The listing builds one solid part. Answer for the finished solid, in the listing's coordinates (mm). Give positions to 0.01 mm unless a question says otherwise; leave off trailing zeros. Order: outer loops, then holes, each group sorted by start corner. A loop starts at its lowest first (then second) coordinate and runs counter-clockwise, first axis right, second up. Notation, with made-up numbers: (-5.75, 81.25) - (4.25, 81.25) arc R13 ccw to (4.25, 94.25) - close; hole circle Ø3 at (-26, 62.5). An arc over 180 degrees is marked (long way). Answer in a Markdown table with one row per item.
from build123d import *

# Parameters (mm, degrees)
SKETCH_1_W      = 260
SKETCH_1_H      = 120
SKETCH_1_R      = 1.8
SKETCH_1_R_2    = 11.5
SKETCH_1_R_3    = 1.75
SKETCH_1_W_2    = 10
SKETCH_1_H_2    = 30.9
SKETCH_1_W_3    = 6
SKETCH_1_H_3    = 6
EXTRUDE_1_DEPTH = 2


with BuildPart() as part:
    # 草圖1 → 填料-伸長1 (new body)
    with BuildSketch(Plane(origin=(0, 0, 0), x_dir=(1, 0, 0), z_dir=(0, 1, 0))):
        Rectangle(SKETCH_1_W, SKETCH_1_H)
        with Locations((-45, -9.55)):
            Circle(SKETCH_1_R, mode=Mode.SUBTRACT)
        with Locations((-45, -40.45)):
            Circle(SKETCH_1_R, mode=Mode.SUBTRACT)
        with Locations((30, -9.55)):
            Circle(SKETCH_1_R, mode=Mode.SUBTRACT)
        with Locations((30, -40.45)):
            Circle(SKETCH_1_R, mode=Mode.SUBTRACT)
        with Locations((95, -25)):
            Circle(SKETCH_1_R_2, mode=Mode.SUBTRACT)
        with Locations((-122, 52)):
            Circle(SKETCH_1_R_3, mode=Mode.SUBTRACT)
        with Locations((-122, -52)):
            Circle(SKETCH_1_R_3, mode=Mode.SUBTRACT)
        with Locations((122, 52)):
            Circle(SKETCH_1_R_3, mode=Mode.SUBTRACT)
        with Locations((122, -52)):
            Circle(SKETCH_1_R_3, mode=Mode.SUBTRACT)
        with Locations((-115, -17.5)):
            Circle(SKETCH_1_R, mode=Mode.SUBTRACT)
        with Locations((-115, -32.5)):
            Circle(SKETCH_1_R, mode=Mode.SUBTRACT)
        with Locations((-70, -25)):
            Rectangle(SKETCH_1_W_2, SKETCH_1_H_2, mode=Mode.SUBTRACT)
        with Locations((55, -50)):
            Rectangle(SKETCH_1_W_3, SKETCH_1_H_3, mode=Mode.SUBTRACT)
        with Locations((55, 0)):
            Rectangle(SKETCH_1_W_3, SKETCH_1_H_3, mode=Mode.SUBTRACT)
        with BuildLine():
            Line((-71.710967932, 42.596685205), (-69.210967932, 42.596685205))
            Line((-69.210967932, 42.596685205), (-69.210967932, 37.901740315))
            ThreePointArc((-69.210967932, 37.901740315), (-70.460967932, 22), (-71.710967932, 37.901740315))
            Line((-71.710967932, 37.901740315), (-71.710967932, 42.596685205))
        make_face(mode=Mode.SUBTRACT)
        with BuildLine():
            Line((-99.710967932, 42.596685205), (-97.210967932, 42.596685205))
            Line((-97.210967932, 42.596685205), (-97.210967932, 37.901740315))
            ThreePointArc((-97.210967932, 37.901740315), (-98.460967932, 22), (-99.710967932, 37.901740315))
            Line((-99.710967932, 37.901740315), (-99.710967932, 42.596685205))
        make_face(mode=Mode.SUBTRACT)
        with BuildLine():
            Line((-43.710967932, 42.596685205), (-41.210967932, 42.596685205))
            Line((-41.210967932, 42.596685205), (-41.210967932, 37.901740315))
            ThreePointArc((-41.210967932, 37.901740315), (-42.460967932, 22), (-43.710967932, 37.901740315))
            Line((-43.710967932, 37.901740315), (-43.710967932, 42.596685205))
        make_face(mode=Mode.SUBTRACT)
        with BuildLine():
            Line((-15.710967932, 42.596685205), (-13.210967932, 42.596685205))
            Line((-13.210967932, 42.596685205), (-13.210967932, 37.901740315))
            ThreePointArc((-13.210967932, 37.901740315), (-14.460967932, 22), (-15.710967932, 37.901740315))
            Line((-15.710967932, 37.901740315), (-15.710967932, 42.596685205))
        make_face(mode=Mode.SUBTRACT)
        with BuildLine():
            Line((12.289032068, 42.596685205), (14.789032068, 42.596685205))
            Line((14.789032068, 42.596685205), (14.789032068, 37.901740315))
            ThreePointArc((14.789032068, 37.901740315), (13.539032068, 22), (12.289032068, 37.901740315))
            Line((12.289032068, 37.901740315), (12.289032068, 42.596685205))
        make_face(mode=Mode.SUBTRACT)
        with BuildLine():
            Line((40.289032068, 42.596685205), (42.789032068, 42.596685205))
            Line((42.789032068, 42.596685205), (42.789032068, 37.901740315))
            ThreePointArc((42.789032068, 37.901740315), (41.539032068, 22), (40.289032068, 37.901740315))
            Line((40.289032068, 37.901740315), (40.289032068, 42.596685205))
        make_face(mode=Mode.SUBTRACT)
        with BuildLine():
            Line((68.289032068, 42.596685205), (70.789032068, 42.596685205))
            Line((70.789032068, 42.596685205), (70.789032068, 37.901740315))
            ThreePointArc((70.789032068, 37.901740315), (69.539032068, 22), (68.289032068, 37.901740315))
            Line((68.289032068, 37.901740315), (68.289032068, 42.596685205))
        make_face(mode=Mode.SUBTRACT)
        with BuildLine():
            Line((96.289032068, 42.596685205), (98.789032068, 42.596685205))
            Line((98.789032068, 42.596685205), (98.789032068, 37.901740315))
            ThreePointArc((98.789032068, 37.901740315), (97.539032068, 22), (96.289032068, 37.901740315))
            Line((96.289032068, 37.901740315), (96.289032068, 42.596685205))
        make_face(mode=Mode.SUBTRACT)
    extrude(amount=EXTRUDE_1_DEPTH)


solid = part.part
Item 1: Consider line 1 (X direction, y = 0.85, z = 52); line 2 (Z direction, x = -115, y = 1.5); line 3 (Z direction, x = -68, y = 0.5). Determine where each line is inside the solid, lowest interval first.
Answer block:
| item | result |
|---|---|
| line 1 | -130 to -123.75, -120.25 to 52, 58 to 120.25, 123.75 to 130 |
| line 2 | -60 to 15.7, 19.3 to 30.7, 34.3 to 60 |
| line 3 | -60 to -37.61, -22.39 to 9.55, 40.45 to 60 |
Item 2: Find section A-A on z = 25. Write down the section's boundary in (x, y).
Answer block:
| item | result |
|---|---|
| outline | (-130, 0) - (-75, 0) - (-75, 2) - (-130, 2) - close; (-65, 0) - (83.5, 0) - (83.5, 2) - (-65, 2) - close; (106.5, 0) - (130, 0) - (130, 2) - (106.5, 2) - close |
Item 3: Determine the mould class of faces 1 (the face through (69.873, 0.986, -22.007)), 2 (the face through (97.873, 0.986, -22.007)), 3 (the face through (-2, 2, -1)) for opening direction Z: pulls with the +Z half, pulls with the -Z half, needs draft (parallel to the pull), parting line crosses it, or undercut.
Answer block:
| item | result |
|---|---|
| face 1 | undercut |
| face 2 | undercut |
| face 3 | needs draft |
Item 4: Find section B-B on z = -30. Count the separate pieces of the cut face and the enclosed holes in it, then the cut area to 3 significant figures.
Answer block:
| item | result |
|---|---|
| separate pieces | 9 |
| enclosed holes | 0 |
| area | 264 mm² |
Item 5: This flat-tipped pin is pushed along its axis until it touches: P1, Ø2, axis at x = -64, z = -13.5, coming from the -Y side. Where does it stop, or does it pass through?
Answer block:
| item | result |
|---|---|
| P1 | y = 0 |
